```python
from build123d import *

# Parameters (mm, degrees)
ESQUISSE1_W             = 52
ESQUISSE1_H             = 17
BOSS_EXTRU_1_DEPTH      = 2
ESQUISSE2_W             = 2
ESQUISSE2_H             = 17
BOSS_EXTRU_2_DEPTH      = 50
ESQUISSE3_R             = 2.5
ENL_V_MAT_EXTRU_1_DEPTH = 50
ESQUISSE4_R             = 2.5
ENL_V_MAT_EXTRU_2_DEPTH = 50


with BuildPart() as part:
    # Esquisse1 → Boss.-Extru.1 (new body)
    with BuildSketch(Plane.XY):
        Rectangle(ESQUISSE1_W, ESQUISSE1_H)
    extrude(amount=BOSS_EXTRU_1_DEPTH)

    # Esquisse2 → Boss.-Extru.2 (add)
    with BuildSketch(Plane.XY.offset(2)):
        with Locations((25, 0)):
            Rectangle(ESQUISSE2_W, ESQUISSE2_H)
    extrude(amount=BOSS_EXTRU_2_DEPTH)

    # Esquisse3 → Enlèv. mat.-Extru.1 (cut)
    with BuildSketch(Plane.XY.offset(2)):
        with Locations((-20, 0)):
            Circle(ESQUISSE3_R)
        with Locations((10, 0)):
            Circle(ESQUISSE3_R)
    extrude(amount=-ENL_V_MAT_EXTRU_1_DEPTH, mode=Mode.SUBTRACT)

    # Esquisse4 → Enlèv. mat.-Extru.2 (cut)
    with BuildSketch(Plane.ZY.offset(-24)):
        with Locations((46, 0)):
            Circle(ESQUISSE4_R)
        with Locations((16, 0)):
            Circle(ESQUISSE4_R)
    extrude(amount=-ENL_V_MAT_EXTRU_2_DEPTH, mode=Mode.SUBTRACT)


solid = part.part
```
The model under review builds one solid part; all positions refer to its coordinate system, in mm. A direction names the side the tool comes from. Round coordinates to 2 decimals unless told otherwise and drop trailing zeros. Loops run counter-clockwise (first coordinate to the right, second up) from the corner with the lowest first, then second, coordinate; pieces in that order, holes last. Notation, with made-up numbers: (4.25, 53.25) -> (10.25, 53.25) arc R22 ccw to (10.25, 76.25) -> close; hole circle Ø3 at (46, 21). An arc over 180 degrees is marked (long way). Answer as a JSON object with one key per item and string values. Group by question number.
1) For faces 5 (the face through (0, 0, 0)), 6 (the face through (24, 0, 27)), list the 3-axis set-ups (+Z, -Z, +X, -X, +Y, -Y) from which the entire face can be reached by the end or side of a thin tool; tool diameter is ignored.
2) For line 1 (Y direction, x = -20, z = 0.9); line 2 (Z direction, x = 7, y = 1.25); line 3 (X direction, y = -4, z = 45.5), list the stretches that pass through material, from the lowest coordinate up. Write a range as [from, to].
3) For pin 1 Ø6 at (x, y) = (-13, -3) entering from +Z; pin 2 Ø2 at (y, z) = (-5.5, 18) entering from -X; pin 3 Ø3 at (x, y) = (10, 0) entering from +Z, all flat-tipped, find the tip position at first contact; note any pin that passes through.
4) We need section A-A on x = 10. Write out the cut boundary in (y, z).
5) We need section D-D on y = 5. Write out the cut boundary in (x, z).
6) We need section C-C on z = 46. Write out the cut boundary in (x, y).
7) We need section B-B on y = 0. Write out the cut boundary in (x, z), then the cut area to 3 significant figures.
8) Mouldability with a two-part tool opening along X and no side actions: class faces 1 (the face through (26, 0, 26)), 2 (the face through (-22.5, 0.1, 1)), 3 (the face through (11, 8.5, 1)), 4 (the face through (7.5, 0.1, 1)) as released by +X, released by -X, zero draft, split by the parting line, or undercut.
Result set:
{
 "1": {"face 5": "-Z, +X, -X, +Y, -Y", "face 6": "+Z, -X, +Y, -Y"},
 "2": {"line 1": "[-8.5, -2.5], [2.5, 8.5]", "line 2": "[0, 2]", "line 3": "[24, 26]"},
 "3": {"pin 1": "z = 2", "pin 2": "x = 24", "pin 3": "through"},
 "4": {"outline": "(-8.5, 0) -> (-2.5, 0) -> (-2.5, 2) -> (-8.5, 2) -> close; (2.5, 0) -> (8.5, 0) -> (8.5, 2) -> (2.5, 2) -> close"},
 "5": {"outline": "(-26, 0) -> (26, 0) -> (26, 52) -> (24, 52) -> (24, 2) -> (-26, 2) -> close"},
 "6": {"outline": "(24, -8.5) -> (26, -8.5) -> (26, -2.5) -> (24, -2.5) -> close; (24, 2.5) -> (26, 2.5) -> (26, 8.5) -> (24, 8.5) -> close"},
 "7": {"outline": "(-26, 0) -> (-22.5, 0) -> (-22.5, 2) -> (-26, 2) -> close; (-17.5, 0) -> (7.5, 0) -> (7.5, 2) -> (-17.5, 2) -> close; (12.5, 0) -> (26, 0) -> (26, 13.5) -> (24, 13.5) -> (24, 2) -> (12.5, 2) -> close; (24, 18.5) -> (26, 18.5) -> (26, 43.5) -> (24, 43.5) -> close; (24, 48.5) -> (26, 48.5) -> (26, 52) -> (24, 52) -> close", "area": "164 mm²"},
 "8": {"face 1": "released by +X", "face 2": "undercut", "face 3": "zero draft", "face 4": "undercut"}
}
